Check sheet for the modelled part. Datum: model origin and axes. Units: mm. Give positions to 0.01 mm unless a question says otherwise; leave off trailing zeros. Write each loop counter-clockwise with the first axis right and the second up, starting at its lowest first coordinate (ties: lowest second). Pieces come first, ordered by that corner, then holes. Notation, with made-up numbers: (50, 67) -> (78, 67) arc R14 ccw to (78, 82) -> close; hole circle Ø9 at (-9.75, 59). An arc over 180 degrees is marked (long way). Answer as a JSON object with one key per item and string values.
Autodesk Inventor part; units mm, degrees
ref_plane "YZ Plane" through (0, 0, 0) normal (1, 0, 0) x (0, 1, 0)
ref_plane "XZ Plane" through (0, 0, 0) normal (0, 1, 0) x (-1, 0, 0)
ref_plane "XY Plane" through (0, 0, 0) normal (0, 0, 1) x (1, 0, 0)
sketch "Sketch1" plane through (0, 0, 0) normal (0, 0, 1) x (1, 0, 0)
  circle A0 centre (0, 0) radius 100
  circle A1 centre (0, 0) radius 160
  dimension "d22" = 200
  dimension "d23" = 320
extrude "Plate1" add sketch "Sketch1" along normal blind 4
sketch "Sketch5" plane through (0, 0, 4) normal (0, 0, 1) x (1, 0, 0)
  circle A0 centre (0, 0) radius 140 construction
  circle A1 centre (0, 140) radius 9
  dimension "d32" = 280
  dimension "d31" = 18
extrude "Cut1" cut sketch "Sketch5" against normal blind 4
pattern_circular "Circular Pattern1" count 8 over 360 about axis through (0, 0, 0) along (0, 0, 1) of "Cut1"
equation "\"d26\" = Thickness"
equation "\"d2\" = Thickness"
equation "\"BendReliefWidth\" = Thickness"
equation "\"BendReliefDepth\" = 0.5 * Thickness"
equation "\"CornerReliefSize\" = 4 * Thickness"
equation "\"MinimumRemnant\" = 2 * Thickness"
equation "\"TransitionRadius\" = BendRadius"
equation "\"JacobiRadiusSize\" = BendRadius"
equation "\"GapSize\" = Thickness"
properties part number "TKS 3108 top DS double flange" material "Stainless Steel"
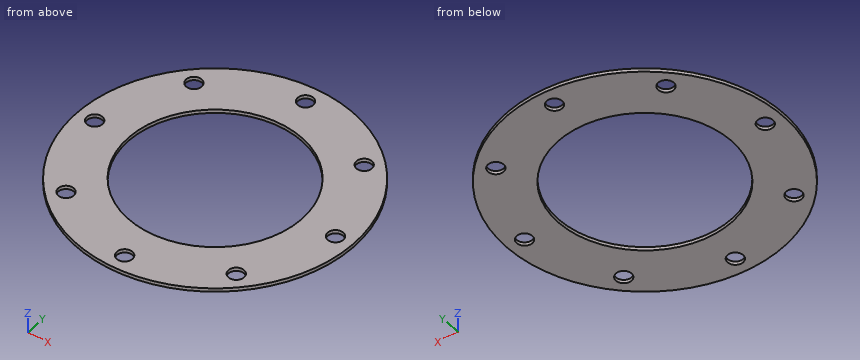
1. Sectioned sample at C-C, the plane x = 140. Enter the section's corners in (y, z).
Determined:
{"outline": "(-77.46, 0) -> (-9, 0) -> (-9, 4) -> (-77.46, 4) -> close; (9, 0) -> (77.46, 0) -> (77.46, 4) -> (9, 4) -> close"}
2. Sectioned sample at A-A, the plane x = 0. Enter the section's corners in (y, z).
Determined:
{"outline": "(-160, 0) -> (-149, 0) -> (-149, 4) -> (-160, 4) -> close; (-131, 0) -> (-100, 0) -> (-100, 4) -> (-131, 4) -> close; (100, 0) -> (131, 0) -> (131, 4) -> (100, 4) -> close; (149, 0) -> (160, 0) -> (160, 4) -> (149, 4) -> close"}
3. Sectioned sample at D-D, the plane z = 2.15. State how many separate pieces and enclosed holes the cut face has, plus the area to 3 significant figures.
Determined:
{"separate pieces": "1", "enclosed holes": "9", "area": "47,000 mm^2"}
4. Go/stop test with flat-tipped pins: P1, Ø20.5, axis at x = 140, y = 0, coming from the -Z side; P2, Ø1.5, axis at x = -103.5, z = 3, coming from the -Y side; P3, Ø1.5, axis at y = 31, z = 2, coming from the -X side; P4, Ø1.5, axis at y = -50, z = 1, coming from the -X side. Record where each tip stops, or that it passes through.
Determined:
{"P1": "z = 0", "P2": "y = -122.65", "P3": "x = -157.11", "P4": "x = -152.23"}
5. Scan lines: L1, parallel to Y at x = 0, z = 1.75; L2, parallel to X at y = 1.5, z = 0.6; L3, parallel to X at y = 105.5, z = 1.15. Record each from-to range of solid material in increasing order. Write a range as [from, to].
Determined:
{"L1": "[-160, -149], [-131, -100], [100, 131], [149, 160]", "L2": "[-159.99, -148.87], [-131.13, -99.99], [99.99, 131.13], [148.87, 159.99]", "L3": "[-120.29, -105.21], [-92.78, 92.78], [105.21, 120.29]"}
